Work out the finished part from the listing and answer in its coordinate system (mm). A direction names the side the tool comes from. Round coordinates to 2 decimals unless told otherwise and drop trailing zeros. Write each loop counter-clockwise with the first axis right and the second up, starting at its lowest first coordinate (ties: lowest second). Pieces come first, ordered by that corner, then holes. Notation, with made-up numbers: (-14.5, -39) -> (-10.5, -39) arc R12 cw to (-10.5, -35) -> close; hole circle Ø11 at (79, 29.5). An arc over 180 degrees is marked (long way). One line per item, written item: value.
```python
from build123d import *

# Parameters (mm, degrees)
F0_W     = 1219.2
F0_H     = 12.7
F1_DEPTH = 406.4
F2_W     = 1219.2
F2_H     = 431.8
F3_DEPTH = 12.7
F4_W     = 203.2
F4_H     = 431.8
F4_W_2   = 127
F5_DEPTH = 330.2
F6_W     = 124.9939593792
F6_H     = 431.8
F7_DEPTH = 254


with BuildPart() as f1:
    # F0 (on Top) → F1 (new body)
    with BuildSketch(Plane.XY):
        with Locations((609.6, 6.35)):
            Rectangle(F0_W, F0_H)
        Polygon((-6.3427571863, 0), (0, 0), (0, 12.7), (0, 444.5), (0, 457.2), (-6.3427571863, 456.896798293), align=None)
        Polygon((1219.2, 12.7), (1219.2, 0), (1243.1888888889, 12.7), align=None)
        Polygon((1219.2, 12.7), (1243.1888888889, 12.7), (1651, 228.6), (1243.1888888889, 444.5), (1219.2, 444.5), align=None)
        with Locations((609.6, 450.85)):
            Rectangle(F0_W, F0_H)
        Polygon((1219.2, 457.2), (1219.2, 444.5), (1243.1888888889, 444.5), align=None)
    extrude(amount=F1_DEPTH)

    # F2 (on face) → F3 (join)
    with BuildSketch(Plane(origin=(0, 0, 0), x_dir=(1, 0, 0), z_dir=(0, 0, -1))):
        with Locations((609.6, -228.6)):
            Rectangle(F2_W, F2_H)
    extrude(amount=-F3_DEPTH)

    # F4 (on face) → F5 (join)
    with BuildSketch(Plane.XY.offset(12.7)):
        with Locations((228.6, 228.6)):
            Rectangle(F4_W, F4_H)
        with Locations((393.7, 228.6)):
            Rectangle(F4_W_2, F4_H)
    extrude(amount=F5_DEPTH)

    # F6 (on face) → F7 (cut)
    with BuildSketch(Plane.XY.offset(342.9)):
        with Locations((394.7030203104, 228.6)):
            Rectangle(F6_W, F6_H)
    extrude(amount=-F7_DEPTH, mode=Mode.SUBTRACT)


solid = f1.part
```
(1) Flat-ended cylindrical pins translate along their axes: pin 1 Ø4 at (y, z) = (171, 53.5) entering from +X; pin 2 Ø3 at (x, y) = (416, 212.5) entering from +Z; pin 3 Ø3 at (y, z) = (131, 174) entering from +X. Find the tip coordinate at first contact, or state that the pin passes through.
Reported:
pin 1: stops at x = 1545.98
pin 2: stops at z = 88.9
pin 3: stops at x = 1469.48
(2) A tool of negligible diameter and unlimited length cuts with its end or side. For faces 1 (the face through (833, 226, 12.7)), 2 (the face through (1432.08, 112.7, 200.36)), from which of +Z, -Z, +X, -X, +Y, -Y can it reach the whole face along a straight path? Write none if from no direction.
Reported:
face 1: +Z
face 2: +Z, -Z, +X, -Y
(3) Find section C-C on z = 378. Give the vertices of the cut face in (x, y), plus the area to 3 significant figures.
Reported:
outline: (-6.34, 0) -> (1219.2, 0) -> (1651, 228.6) -> (1219.2, 457.2) -> (0, 457.2) -> (-6.34, 456.9) -> close; hole (0, 12.7) -> (1219.2, 12.7) -> (1219.2, 444.5) -> (0, 444.5) -> close
area: 133,000 mm2
(4) Find section D-D on x = 198. Give the vertices of the cut face in (y, z).
Reported:
outline: (0, 0) -> (457.2, 0) -> (457.2, 406.4) -> (444.5, 406.4) -> (444.5, 342.9) -> (12.7, 342.9) -> (12.7, 406.4) -> (0, 406.4) -> close
(5) Consider probe 1 along Y at (x, z) = (954.5, 156.5); probe 2 along X at (y, z) = (418.5, 20); probe 3 along X at (y, z) = (21, 293). Determine where each line is inside the solid, lowest interval first.
Reported:
probe 1: y = 0 to 12.7, 444.5 to 457.2
probe 2: x = -6.34 to 0, 127 to 457.2, 1219.2 to 1292.3
probe 3: x = -6.34 to 0, 127 to 332.21, 1219.2 to 1258.87
(6) Find section B-B on y = 112.5. Give the vertices of the cut face in (x, z).
Reported:
outline: (-6.34, 0) -> (1431.7, 0) -> (1431.7, 406.4) -> (1219.2, 406.4) -> (1219.2, 12.7) -> (457.2, 12.7) -> (457.2, 88.9) -> (332.21, 88.9) -> (332.21, 342.9) -> (127, 342.9) -> (127, 12.7) -> (0, 12.7) -> (0, 406.4) -> (-6.34, 406.4) -> close
(7) For a pull along X with two mould halves and no side action, classify faces 3 (the face through (228, 232, 342.9)), 4 (the face through (127, 226, 175)), 5 (the face through (-6.343, 232, 200)), 6 (the face through (1438.12, 341.3, 200.36)) as pulls with the +X half, pulls with the -X half, needs draft (parallel to the pull), parting line crosses it, or undercut.
Reported:
face 3: undercut
face 4: undercut
face 5: pulls with the -X half
face 6: pulls with the +X half
(8) Find section A-A on z = 139. Give the vertices of the cut face in (x, y).
Reported:
outline: (-6.34, 0) -> (1219.2, 0) -> (1651, 228.6) -> (1219.2, 457.2) -> (0, 457.2) -> (-6.34, 456.9) -> close; hole (0, 12.7) -> (127, 12.7) -> (127, 444.5) -> (0, 444.5) -> close; hole (332.21, 12.7) -> (1219.2, 12.7) -> (1219.2, 444.5) -> (332.21, 444.5) -> close
